Part model, mm, in its own coordinate system. Face numbers are marked on the shaded views. A direction names the side the tool comes from. Round coordinates to 2 decimals unless told otherwise and drop trailing zeros. Loops run counter-clockwise (first coordinate to the right, second up) from the corner with the lowest first, then second, coordinate; pieces in that order, holes last. Notation, with made-up numbers: M 39.25,84.25 L 65.25,84.25 A21 ccw 65.25,121.25 Z; hole C -3,13 d6. An arc over 180 degrees is marked long. Answer as CSV lines item,"result". Start each with the question number.
Item 1: Drop flat-ended pins along their axis: pin 1 Ø1 at (y, z) = (27, 5) entering from +X; pin 2 Ø6 at (x, y) = (-8.5, -14.5) entering from +Z. Give the stop position or say it passes through.
Item 2: Band-saw the part on A-A (x = -38.5). Count the separate pieces of the cut face and the enclosed holes in it, and give its area (3 significant figures).
Item 3: Band-saw the part on D-D (x = -9.5). Give the cut face in (y, z), and give its area (4 significant figures).
Item 4: Wall check: line 1 (X direction, y = -26.5, z = 4.25); line 2 (Y direction, x = 38.5, z = 4.7); line 3 (X direction, y = 26.5, z = 4.1). Give the ranges that are in metal, low to high.
Item 5: Band-saw the part on C-C (z = 4.4). Give the cut face in (x, y), and give its area (3 significant figures).
Item 6: Which spindle directions (+Z, -Z, +X, -X, +Y, -Y) get a long thin tool onto all of the face, cutting with end or side? Do the marked faces 1 and 2. Say none if no direction does.
Autodesk Inventor part; units mm, degrees
ref_plane "YZ Plane" through (0, 0, 0) normal (1, 0, 0) x (0, 1, 0)
ref_plane "XZ Plane" through (0, 0, 0) normal (0, 1, 0) x (-1, 0, 0)
ref_plane "XY Plane" through (0, 0, 0) normal (0, 0, 1) x (1, 0, 0)
sketch "Sketch1" plane through (0, 0, 0) normal (0, 0, 1) x (1, 0, 0)
  line L0 (-45, 37) -> (45, 37)
  line L1 (45, 37) -> (45, -37)
  line L2 (45, -37) -> (-45, -37)
  line L3 (-45, -37) -> (-45, 37)
  line L4 (-38.5, 26.5) -> (38.5, 26.5) construction
  line L5 (38.5, 26.5) -> (38.5, -26.5) construction
  line L6 (38.5, -26.5) -> (-38.5, -26.5) construction
  line L7 (-38.5, -26.5) -> (-38.5, 26.5) construction
  circle A0 centre (-38.5, 26.5) radius 2.5
  circle A1 centre (38.5, 26.5) radius 2.5
  circle A2 centre (38.5, -26.5) radius 2.5
  circle A3 centre (-38.5, -26.5) radius 2.5
  point P0 (0, 0)
  point P1 (45, 0)
  point P2 (0, 37)
  point P3 (38.5, 0)
  point P4 (0, 26.5)
  dimension "d0" = 90
  dimension "d1" = 74
  dimension "d2" = 77
  dimension "d3" = 53
  dimension "d14" = 5
extrude "Extrusion1" add sketch "Sketch1" along normal blind 3 contours L0 L1 L2 L3 | A0 | A1 | A2 | A3
extrude "Extrusion2" add sketch "Sketch1" along normal blind 6 contours A0 | A1 | A2 | A3
chamfer "Chamfer1" distance 3 angle 45 4 edges at (-41, 26.5, 3) (36, 26.5, 3) (36, -26.5, 3) (-41, -26.5, 3)
hole "Hole1" at (38.5, 26.5, 0) at (38.5, -26.5, 0) at (-38.5, -26.5, 0) at (-38.5, 26.5, 0) direction (0, 0, 1) diameter 3.3 end through all
fillet "Fillet1" radius 5 4 edges at (45, 37, 1.5) (45, -37, 1.5) (-45, -37, 1.5) (-45, 37, 1.5)
chamfer "Chamfer2" distance 0.5 angle 45 9 edges at (0, 37, 0) (-43.5355, 35.5355, 0) (-45, 0, 0) (-43.5355, -35.5355, 0) (0, -37, 0) (43.5355, -35.5355, 0) (45, 0, 0) (43.5355, 35.5355, 0) (0, 37, 3)
equation "\"d0\" = length"
equation "\"d1\" = width"
equation "\"d4\" = thickness"
equation "\"d15\" = thickness + bump"
equation "\"width\" = 74"
equation "\"length\" = 90"
equation "\"thickness\" = 3"
equation "\"bump\" = 3"
properties part number "temp-logger-base-plate" material "ABS Plastic"
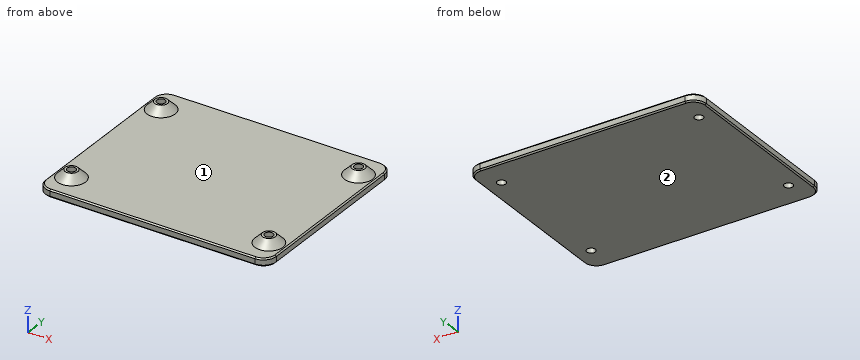
Answer block:
1,pin 1,"stops at x = 42.47"
1,pin 2,"stops at z = 3"
2,separate pieces,"3"
2,enclosed holes,"0"
2,area,"230 mm^2"
3,outline,"M -37,0.5 L -36.5,0 L 36.5,0 L 37,0.5 L 37,2.5 L 36.5,3 L -36.5,3 L -37,2.5 Z"
3,area,"221.5 mm^2"
4,line 1,"x = -42.75 to -40.15, -36.85 to -34.25, 34.25 to 36.85, 40.15 to 42.75"
4,line 2,"y = -30.3 to -28.15, -24.85 to -22.7, 22.7 to 24.85, 28.15 to 30.3"
4,line 3,"x = -42.9 to -40.15, -36.85 to -34.1, 34.1 to 36.85, 40.15 to 42.9"
5,outline,"C -38.5,-26.5 d8.2; C -38.5,26.5 d8.2; C 38.5,-26.5 d8.2; C 38.5,26.5 d8.2; hole C -38.5,-26.5 d3.3; hole C -38.5,26.5 d3.3; hole C 38.5,-26.5 d3.3; hole C 38.5,26.5 d3.3"
5,area,"177 mm^2"
6,face 1,"+Z"
6,face 2,"-Z, +X, -X, +Y, -Y"
